Build history of the part. All positions in model axes, mm. A direction names the side the tool comes from. Round coordinates to 2 decimals unless told otherwise and drop trailing zeros. Loops run counter-clockwise (first coordinate to the right, second up) from the corner with the lowest first, then second, coordinate; pieces in that order, holes last. Notation, with made-up numbers: (82.25, 55.25) - (124.25, 55.25) arc R15 ccw to (124.25, 60.25) - close; hole circle Ø10 at (-12.75, 61). An arc over 180 degrees is marked (long way). Use one line per item in the form item = value. Start each with the question number.
Q1. Saw through at B-B (x = 2.75). Give the cut face in (y, z).
Q2. Saw through at A-A (z = 0). Give the cut face in (x, y).
Q3. Saw through at C-C (y = 5.5). Give the cut face in (x, z), then the cut area to 3 significant figures.
Q4. 3-axis set-ups, long thin cutter, end or side, ignore diameter. For faces 4 (the face through (0, 20, 0)), 5 (the face through (-2.87, 9.86, 2.64)), 6 (the face through (2.192, -4.944, -4.214)): which of +Z, -Z, +X, -X, +Y, -Y reach the whole face in a straight line?
Q5. Mould opens along X. For faces 1 (the face through (-0.29, -2.86, 2.23)), 2 (the face through (-5.994, -0.493, 0.264)), 3 (the face through (2, -13, -2)) say: released by +X, released by -X, zero draft, split by the parting line, or undercut.
Q6. Saw through at D-D (x = 0). Give the cut face in (y, z), then the cut area to 3 significant figures.
Q7. Drill centre lines: line 1 (Z direction, x = 0, y = -2.5); line 2 (Y direction, x = 3.25, z = -5); line 3 (X direction, y = 2, z = -1.5). Where is each one in solid material? Low to high.
Q8. Pin check, flat tips, straight feed: pin 1 (1.5 mm diameter, centred on x = 4, y = 12, fed in from +Z); pin 2 (2 mm diameter, centred on y = 2, z = 3.5, fed in from -X); pin 3 (5 mm diameter, centred on y = 16, z = 1, fed in from -X). Stop position of each tip, or through.
```python
from build123d import *

# Parameters (mm, degrees)
F0_R     = 3.9
F0_R_2   = 2.25
F1_DEPTH = 13
F0_R_3   = 4.75
F3_DEPTH = 9
F0_R_4   = 6
F4_DEPTH = 1
F5_DEPTH = 20
F6_DEPTH = 7


with BuildPart() as f1:
    # F0 (on Front) → F1 (new body)
    with BuildSketch(Plane.XZ):
        Circle(F0_R)
        Circle(F0_R_2, mode=Mode.SUBTRACT)
    extrude(amount=F1_DEPTH)

    # F0 (on Front) → F3 (join)
    with BuildSketch(Plane.XZ):
        Circle(F0_R_3)
        Circle(F0_R, mode=Mode.SUBTRACT)
    extrude(amount=F3_DEPTH)

    # F0 (on Front) → F4 (join)
    with BuildSketch(Plane.XZ):
        Circle(F0_R_4)
        Circle(F0_R_3, mode=Mode.SUBTRACT)
    extrude(amount=F4_DEPTH)

    # F0 (on Front) → F5 (join)
    with BuildSketch(Plane.XZ):
        Circle(F0_R)
        Circle(F0_R_2, mode=Mode.SUBTRACT)
        Circle(F0_R_2)
    extrude(amount=-F5_DEPTH)

    # F0 (on Front) → F6 (cut)
    with BuildSketch(Plane.XZ):
        Circle(F0_R_2)
    extrude(amount=-F6_DEPTH, mode=Mode.SUBTRACT)


solid = f1.part
```
Report:
q1.outline = (-13, -2.77) - (-9, -2.77) - (-9, -3.87) - (-1, -3.87) - (-1, -5.33) - (0, -5.33) - (0, -2.77) - (20, -2.77) - (20, 2.77) - (0, 2.77) - (0, 5.33) - (-1, 5.33) - (-1, 3.87) - (-9, 3.87) - (-9, 2.77) - (-13, 2.77) - close
q2.outline = (-6, -1) - (-4.75, -1) - (-4.75, -9) - (-3.9, -9) - (-3.9, -13) - (-2.25, -13) - (-2.25, 7) - (2.25, 7) - (2.25, -13) - (3.9, -13) - (3.9, -9) - (4.75, -9) - (4.75, -1) - (6, -1) - (6, 0) - (3.9, 0) - (3.9, 20) - (-3.9, 20) - (-3.9, 0) - (-6, 0) - close
q3.outline = circle Ø7.8 at (0, 0); hole circle Ø4.5 at (0, 0)
q3.area = 31.9 mm²
q4.face_4 = +Z, -Z, +X, -X, +Y
q4.face_5 = +Y
q4.face_6 = -Y
q5.face_1 = undercut
q5.face_2 = split by the parting line
q5.face_3 = zero draft
q6.outline = (-13, -3.9) - (-9, -3.9) - (-9, -4.75) - (-1, -4.75) - (-1, -6) - (0, -6) - (0, -3.9) - (20, -3.9) - (20, 3.9) - (0, 3.9) - (0, 6) - (-1, 6) - (-1, 4.75) - (-9, 4.75) - (-9, 3.9) - (-13, 3.9) - (-13, 2.25) - (7, 2.25) - (7, -2.25) - (-13, -2.25) - close
q6.area = 185 mm²
q7.line_1 = -4.75 to -2.25, 2.25 to 4.75
q7.line_2 = -1 to 0
q7.line_3 = -3.6 to -1.68, 1.68 to 3.6
q8.pin_1 = 2.16
q8.pin_2 = -2.99
q8.pin_3 = -3.9
